Verification items for the finished model (mm, model axes). Face numbers are marked on the shaded views. A direction names the side the tool comes from. Give positions to 0.01 mm unless a question says otherwise; leave off trailing zeros. Order: outer loops, then holes, each group sorted by start corner. A loop starts at its lowest first (then second) coordinate and runs counter-clockwise, first axis right, second up. Notation, with made-up numbers: (86, 56.25) -> (119, 56.25) arc R18 ccw to (119, 65.25) -> close; hole circle Ø11 at (30.5, 0.25). An arc over 180 degrees is marked (long way). Return JSON: item names as keys, results as strings. Group by question number.
(1) Release check for a two-part mould opening along X. For the marked faces 1, 2 and 3 record: pulls with the +X half, pulls with the -X half, needs draft (parallel to the pull), parting line crosses it, or undercut.
(2) Thickness scan on line 1 along X through (y, z) = (-78, -10.5); line 2 along X through (y, z) = (-42, 19.5); line 3 along Z through (x, y) = (34, -22). Record the ranges inside material, lowest first.
(3) Cross-section at C-C on x = -2. Enter the section's corners in (y, z).
(4) Tool access check on the marked faces 4, 5, 6 and 7. Record the directions out of +Z, -Z, +X, -X, +Y, -Y that give a thin tool (end or side, any length) a straight path to the whole face; none if there is none.
(5) Cross-section at B-B on z = -48. Enter the section's corners in (x, y), then the cut area to 3 significant figures.
(6) Cross-section at A-A on y = -76. Enter the section's corners in (x, z), then the cut area to 3 significant figures.
(7) Depth check by flat-ended pin: pin 1 Ø2.5 at (x, z) = (-113.5, 1.5) entering from +Y; pin 2 Ø1.7 at (x, y) = (-102, -30) entering from +Z; pin 3 Ø21 at (y, z) = (-79, 0) entering from +X; pin 4 Ø12 at (x, z) = (64, -31) entering from +Y. Enter the tip coordinate at first touch or a pass-through.
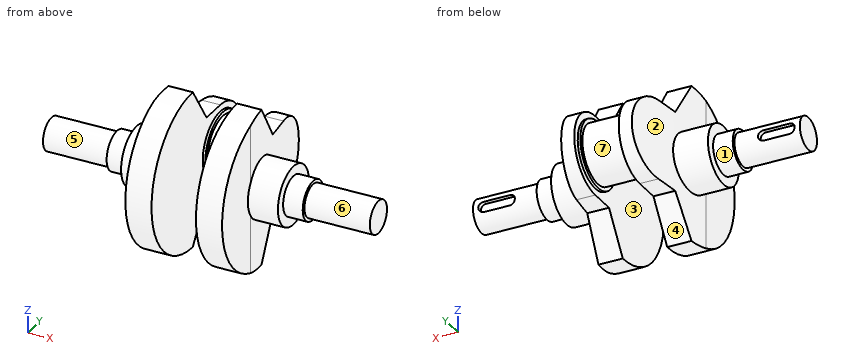
from build123d import *

# Parameters (mm, degrees)
SKETCH1_R           = 22.5
BOSS_EXTRUDE1_DEPTH = 15
SKETCH2_R           = 25.5
BOSS_EXTRUDE2_DEPTH = 2
BOSS_EXTRUDE3_DEPTH = 20
CUT_EXTRUDE1_DEPTH  = 99
BOSS_EXTRUDE4_REACH = 77
SKETCH5_R           = 22.5
SKETCH6_R           = 15
BOSS_EXTRUDE5_DEPTH = 15
SKETCH7_R           = 12.5
BOSS_EXTRUDE6_DEPTH = 50
CUT_EXTRUDE2_DEPTH  = 4


with BuildPart() as part:
    # Sketch1 → Boss-Extrude1 (new body, symmetric)
    with BuildSketch(Plane(origin=(0, 0, 0), x_dir=(0, 0, -1), z_dir=(1, 0, 0))):
        Circle(SKETCH1_R)
    extrude(amount=BOSS_EXTRUDE1_DEPTH, both=True)

    # Sketch2 → Boss-Extrude2 (add)
    with BuildSketch(Plane(origin=(15, 0, 0), x_dir=(0, 0, -1), z_dir=(1, 0, 0))):
        Circle(SKETCH2_R)
    extrude(amount=BOSS_EXTRUDE2_DEPTH)

    # Sketch3 → Boss-Extrude3 (add)
    with BuildSketch(Plane(origin=(17, 0, 0), x_dir=(0, 0, -1), z_dir=(1, 0, 0))):
        with BuildLine():
            Line((-30.5, 0), (-30.5, -20))
            Line((-30.5, -20), (-60, -40))
            ThreePointArc((-60, -40), (0, -100), (60, -40))
            Line((60, -40), (30.5, -20))
            Line((30.5, -20), (30.5, 0))
            ThreePointArc((30.5, 0), (0, 30.5), (-30.5, 0))
        make_face()
    extrude(amount=BOSS_EXTRUDE3_DEPTH)

    # Sketch4 → Cut-Extrude1 (cut, symmetric)
    with BuildSketch(Plane.XY):
        with BuildLine():
            Line((27, 30.5), (37, 30.5))
            Line((37, 30.5), (37, -58.5))
            ThreePointArc((37, -58.5), (32.963579083, -13.891732687), (27, 30.5))
        make_face()
    extrude(amount=CUT_EXTRUDE1_DEPTH, both=True, mode=Mode.SUBTRACT)

    # Sketch5 → Boss-Extrude4 (add, up to next)
    with BuildSketch(Plane(origin=(60, 0, 0), x_dir=(0, 0, -1), z_dir=(1, 0, 0)), mode=Mode.PRIVATE) as boss_extrude4_sk1:
        with Locations((0, -40)):
            Circle(SKETCH5_R)
    boss_extrude4_tool1 = extrude(boss_extrude4_sk1.sketch, amount=-BOSS_EXTRUDE4_REACH, mode=Mode.PRIVATE) - part.part
    add(boss_extrude4_tool1.solids().sort_by_distance((60, -40, 0))[0])

    # Sketch6 → Boss-Extrude5 (add)
    with BuildSketch(Plane(origin=(60, 0, 0), x_dir=(0, 0, -1), z_dir=(1, 0, 0))):
        with Locations((0, -40)):
            Circle(SKETCH6_R)
    extrude(amount=BOSS_EXTRUDE5_DEPTH)

    # Sketch7 → Boss-Extrude6 (add)
    with BuildSketch(Plane(origin=(75, 0, 0), x_dir=(0, 0, -1), z_dir=(1, 0, 0))):
        with Locations((0, -40)):
            Circle(SKETCH7_R)
    extrude(amount=BOSS_EXTRUDE6_DEPTH)

    # Sketch9 → Cut-Extrude2 (cut)
    with BuildSketch(Plane(origin=(0, -27.5, 0), x_dir=(-1, 0, 0), z_dir=(0, 1, 0))):
        with BuildLine():
            Line((-97, -4), (-117, -4))
            ThreePointArc((-117, -4), (-121, 0), (-117, 4))
            Line((-117, 4), (-97, 4))
            ThreePointArc((-97, 4), (-93, 0), (-97, -4))
        make_face()
    extrude(amount=-CUT_EXTRUDE2_DEPTH, mode=Mode.SUBTRACT)

    # Mirror2: part across plane


with BuildPart() as part_1:
    add(part.part)
    add(part.part.mirror(Plane(origin=(0, 0, 0), x_dir=(0, 0, 1), z_dir=(1, 0, 0))))


solid = part_1.part
Verdict:
{
 "1": {"face 1": "needs draft", "face 2": "pulls with the -X half", "face 3": "undercut"},
 "2": {"line 1": "-37 to -17, 17 to 37", "line 2": "-60 to -17, 17 to 60", "line 3": "-13.5 to 13.5"},
 "3": {"outline": "circle Ø45 at (0, 0)"},
 "4": {"face 4": "-Z, +X, -X, +Y", "face 5": "-X", "face 6": "+X", "face 7": "none"},
 "5": {"outline": "(-37, -76) -> (-17, -76) -> (-17, -31.86) -> (-34.82, -31.86) arc R1034.5 ccw to (-37, -58.5) -> close; (17, -76) -> (37, -76) -> (37, -58.5) arc R1034.5 ccw to (34.82, -31.86) -> (17, -31.86) -> close", "area": "1,710 mm²"},
 "6": {"outline": "(-37, -48) -> (-17, -48) -> (-17, 48) -> (-37, 48) -> close; (17, -48) -> (37, -48) -> (37, 48) -> (17, 48) -> close", "area": "3,840 mm²"},
 "7": {"pin 1": "y = -31.5", "pin 2": "z = 8.52", "pin 3": "x = 37", "pin 4": "through"}
}
